Can you work these out from the drawing? Everything is in mm from the part's minimum corner. A direction names the side the tool comes from. Coordinates: 2 decimals unless noted, no trailing zeros. Write each loop counter-clockwise with the first axis right and the second up, starting at its lowest first coordinate (ties: lowest second). Pieces come first, ordered by that corner, then holes.
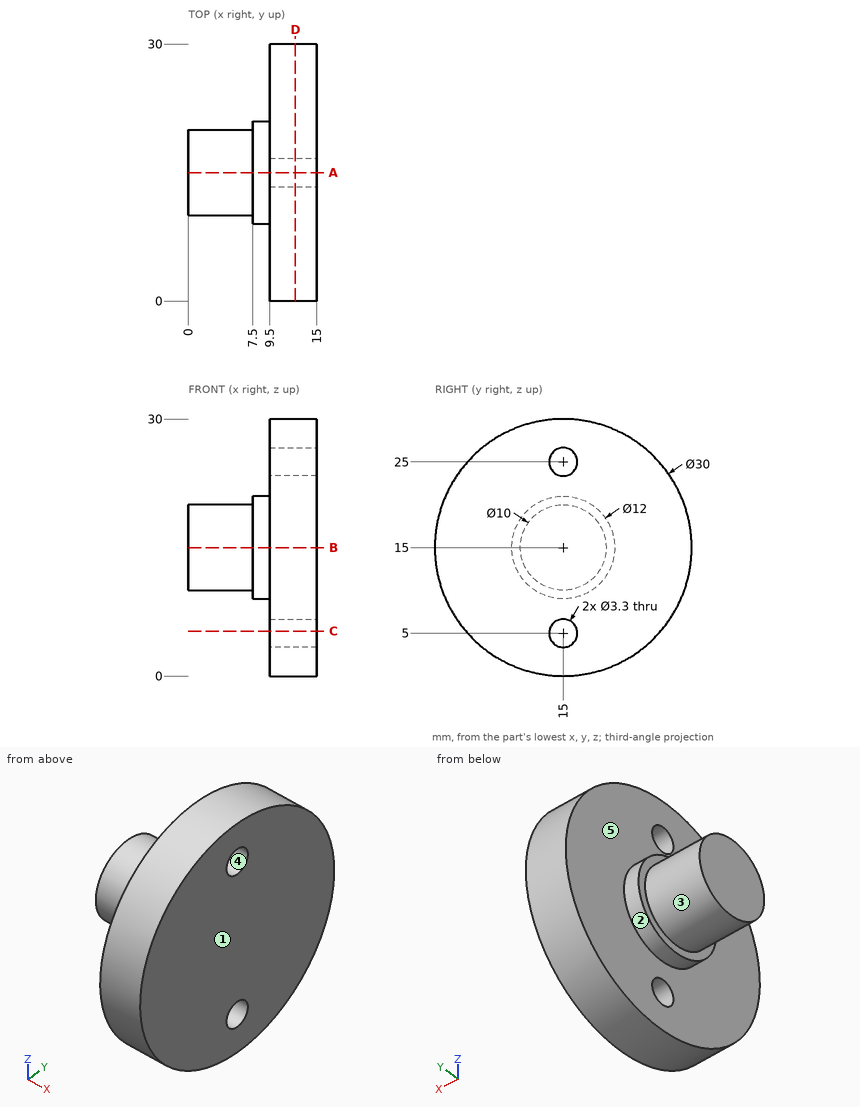
1. If I drill on line 1 (X direction, y = 28, z = 14.75); line 2 (Y direction, x = 11.95, z = 5); line 3 (Y direction, x = 9.75, z = 4.25), over which ranges is the centre line in solid material (lowest first)?
2. I want a section at B-B (z = 15). List the corners of the cut face in (x, y) for me.
3. Thinking about a two-plate mould opening in Z: for the marked faces 3, 4 and 5, which applies, pulls with the +Z half, pulls with the -Z half, needs draft (parallel to the pull), parting line crosses it, or undercut?
4. I want a section at C-C (z = 5.25). List the corners of the cut face in (x, y) for me.
5. On a 3-axis mill with a long thin cutter (end or side, diameter ignored), from which of +Z, -Z, +X, -X, +Y, -Y can I reach the whole of each face in a straight line? I mean the marked faces 1 and 2. Say none if no direction works.
6. I want a section at D-D (x = 12.5). List the corners of the cut face in (y, z) for me, then the cut area to 3 significant figures.
7. I want a section at A-A (y = 15). List the corners of the cut face in (x, z) for me, then the cut area to 3 significant figures.
8. For pin 1 Ø4 at (x, y) = (6.5, 19.5) entering from +Z; pin 2 Ø2 at (y, z) = (6, 13.5) entering from -X; pin 3 Ø6 at (x, z) = (4.5, 20.5) entering from +Y, each with a flat end and sliding along its axis, tell me the tip position at first contact or that it passes through.
Response values:
1. line 1: x = 9.5 to 15
1. line 2: y = 3.82 to 13.35, 16.65 to 26.18
1. line 3: y = 4.54 to 13.53, 16.47 to 25.46
2. outline: (0, 10) - (7.5, 10) - (7.5, 9) - (9.5, 9) - (9.5, 0) - (15, 0) - (15, 30) - (9.5, 30) - (9.5, 21) - (7.5, 21) - (7.5, 20) - (0, 20) - close
3. face 3: parting line crosses it
3. face 4: undercut
3. face 5: needs draft
4. outline: (9.5, 3.6) - (15, 3.6) - (15, 13.37) - (9.5, 13.37) - close; (9.5, 16.63) - (15, 16.63) - (15, 26.4) - (9.5, 26.4) - close
5. face 1: +Z, -Z, +X, +Y, -Y
5. face 2: -X
6. outline: circle Ø30 at (15, 15); hole circle Ø3.3 at (15, 5); hole circle Ø3.3 at (15, 25)
6. area: 690 mm2
7. outline: (0, 10) - (7.5, 10) - (7.5, 9) - (9.5, 9) - (9.5, 6.65) - (15, 6.65) - (15, 23.35) - (9.5, 23.35) - (9.5, 21) - (7.5, 21) - (7.5, 20) - (0, 20) - close; (9.5, 0) - (15, 0) - (15, 3.35) - (9.5, 3.35) - close; (9.5, 26.65) - (15, 26.65) - (15, 30) - (9.5, 30) - close
7. area: 228 mm2
8. pin 1: stops at z = 20.32
8. pin 2: stops at x = 9.5
8. pin 3: stops at y = 19.33
